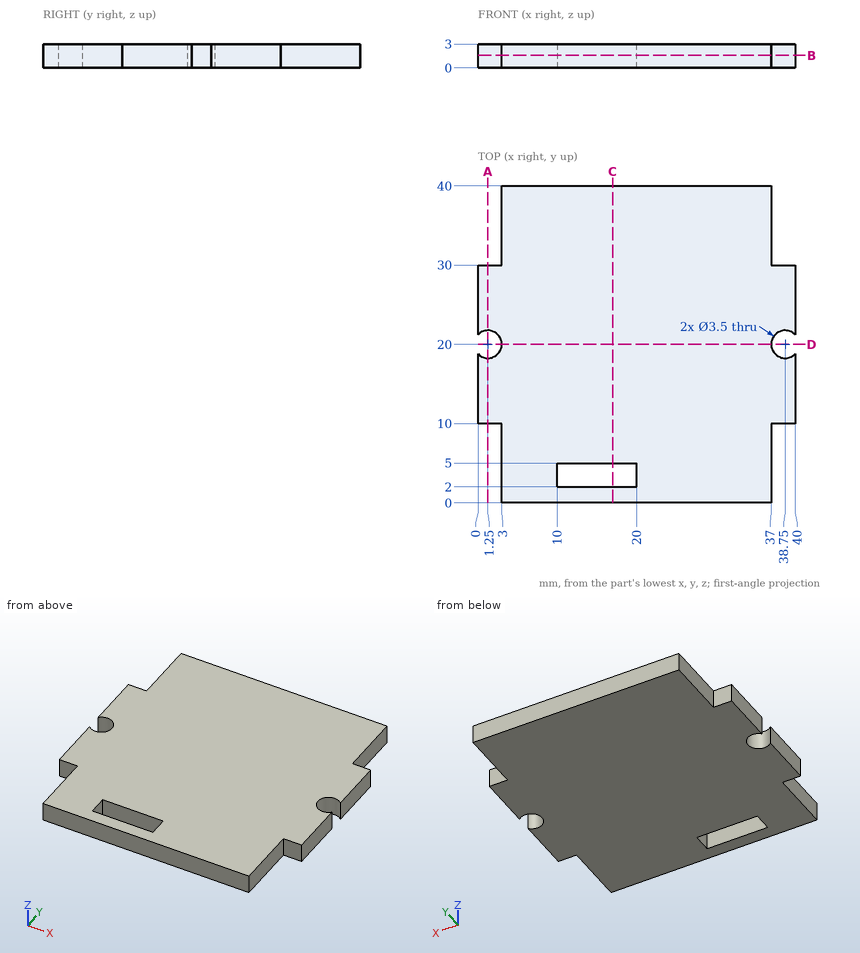
The drawing under review shows one solid part. Ordinate dimensions are in mm from its lowest x, y, z. Round coordinates to 2 decimals unless told otherwise and drop trailing zeros. Write each loop counter-clockwise with the first axis right and the second up, starting at its lowest first coordinate (ties: lowest second). Pieces come first, ordered by that corner, then holes. Notation, with made-up numbers: (-0.5, -9.75) - (45.5, -9.75) arc R19 ccw to (45.5, 6.25) - close; hole circle Ø11 at (-39.75, 42.25). An arc over 180 degrees is marked (long way). Use a Markdown table: item, result. Add a question column.
1. We need section B-B (z = 1.55). State the section outline as (x, y) points, then the cut area to 3 significant figures.
2. Wall thickness on probe 1 along Y at (x, z) = (38.75, 0.8); probe 2 along Y at (x, z) = (12, 0.75); probe 3 along X at (y, z) = (36, 1.55): over which ranges is each line inside the solid? List them lowest first.
3. We need section D-D (y = 20). State the section outline as (x, z) points, then the cut area to 3 significant figures.
4. We need section A-A (x = 1.25). State the section outline as (y, z) points, then the cut area to 3 significant figures.
5. Clearance check with flat-ended pins moving along their axes: pin 1 (0.9 mm diameter, centred on x = 1.5, z = 1, fed in from +Y); pin 2 (0.9 mm diameter, centred on y = 33, z = 1, fed in from +X); pin 3 (3 mm diameter, centred on x = 38.75, y = 20, fed in from +Z); pin 4 (1.5 mm diameter, centred on x = 2, z = 1, fed in from -Y). State where each tip first meets the part, or that it passes through.
6. We need section C-C (x = 17). State the section outline as (y, z) points.
Output:
| question | item | result |
|---|---|---|
| 1 | outline | (0, 10) - (3, 10) - (3, 0) - (37, 0) - (37, 10) - (40, 10) - (40, 18.78) arc R1.75 cw (long way) to (40, 21.22) - (40, 30) - (37, 30) - (37, 40) - (3, 40) - (3, 30) - (0, 30) - (0, 21.22) arc R1.75 cw (long way) to (0, 18.78) - close; hole (10, 2) - (20, 2) - (20, 5) - (10, 5) - close |
| 1 | area | 1,430 mm2 |
| 2 | probe 1 | y = 10 to 18.25, 21.75 to 30 |
| 2 | probe 2 | y = 0 to 2, 5 to 40 |
| 2 | probe 3 | x = 3 to 37 |
| 3 | outline | (3, 0) - (37, 0) - (37, 3) - (3, 3) - close |
| 3 | area | 102 mm2 |
| 4 | outline | (10, 0) - (18.25, 0) - (18.25, 3) - (10, 3) - close; (21.75, 0) - (30, 0) - (30, 3) - (21.75, 3) - close |
| 4 | area | 49.5 mm2 |
| 5 | pin 1 | stops at y = 30 |
| 5 | pin 2 | stops at x = 37 |
| 5 | pin 3 | passes through |
| 5 | pin 4 | stops at y = 10 |
| 6 | outline | (0, 0) - (2, 0) - (2, 3) - (0, 3) - close; (5, 0) - (40, 0) - (40, 3) - (5, 3) - close |
